Work out the finished part from the listing and answer in its coordinate system (mm). A direction names the side the tool comes from. Round coordinates to 2 decimals unless told otherwise and drop trailing zeros. Write each loop counter-clockwise with the first axis right and the second up, starting at its lowest first coordinate (ties: lowest second). Pieces come first, ordered by that corner, then holes.
1. Find section A-A (y = 0). Write down the section's boundary in (x, z), and give its area (3 significant figures).
2. Straight lines are drawn through the part: probe 1 along Y at (x, z) = (1.5, 0); probe 2 along Y at (x, z) = (0.5, -1); probe 3 along Y at (x, z) = (3.75, 0.25). For each, find the intervals that lie inside material, in ascending order.
3. Flat-ended cylindrical pins translate along their axes: pin 1 Ø2 at (x, y) = (1.5, 5.5) entering from +Z; pin 2 Ø7.5 at (y, z) = (16, -0.5) entering from -X; pin 3 Ø2 at (x, y) = (-0.5, 42) entering from -Z. Find the tip coordinate at first contact, or state that the pin passes through.
4. A tool of negligible diameter and unlimited length cuts with its end or side. For faces 3 (the face through (4, -2, -6)), 4 (the face through (-1, 20, 0)), 5 (the face through (1.8, 23.2, 3.4)), 6 (the face through (0.043, 22.839, 4.435)), 7 (the face through (0.043, 22.357, -4.476)), from which of +Z, -Z, +X, -X, +Y, -Y can it reach the whole face along a straight path? Write none if from no direction.
5. Determine the mould class of faces 1 (the face through (-1.5, 38, 0)), 2 (the face through (-4, -2, -6)) for opening direction Y: pulls with the +Y half, pulls with the -Y half, needs draft (parallel to the pull), parting line crosses it, or undercut.
6. Find section C-C (y = 21.5). Write down the section's boundary in (x, z), and give its area (3 significant figures).
7. Find section B-B (z = -1.5). Count the separate pieces of the cut face and the enclosed holes in it, and give its area (3 significant figures).
```python
from build123d import *

# Parameters (mm, degrees)
BOSS_EXTRU_1_START      = -2.0000001
BOSS_EXTRU_1_DEPTH      = 2.0000001
BOSS_EXTRU_1_START_2    = 2.0000001
BOSS_EXTRU_1_2_DEPTH    = 1.088880676
BOSS_EXTRU_1_START_3    = 3.256370695
BOSS_EXTRU_1_3_DEPTH    = 1.743629305
BOSS_EXTRU_1_START_4    = 3.172268194
BOSS_EXTRU_1_4_DEPTH    = 0.084102501
ENL_V_MAT_EXTRU_1_DEPTH = 9


with BuildPart() as part:
    # Esquisse2 → Révolution1 (revolve)
    with BuildSketch(Plane.XY, mode=Mode.PRIVATE) as r_volution1_sk:
        Polygon((2.4e-16, 6), (4, 6), (4, 7), (2.9999999999999996, 8), (-1.8e-16, 8), align=None)
    revolve(r_volution1_sk.sketch.rotate(Axis((0, 0, 0), (1, 0, 0)), 90), axis=Axis((0, 0, 0), (1, 0, 0)))



with BuildPart() as body_2:
    # Esquisse3 → Révolution2 (revolve)
    with BuildSketch(Plane.XY, mode=Mode.PRIVATE) as r_volution2_sk:
        Polygon((0, 48.99999999999999), (4.01e-15, 51), (2, 51), (4, 49.99999999999999), (4, 48.99999999999999), align=None)
    revolve(r_volution2_sk.sketch.rotate(Axis((0, 45, 0), (1, 0, 0)), 90), axis=Axis((0, 45, 0), (1, 0, 0)))


with BuildPart() as part_1:
    add(part.part)

    add(body_2.part)  # Boss.-Extru.1 merges body 2
    # Boss.-Extru.1: read off the stored shape, not the designer's step
    # Boss.-Extru.1 outline → Boss.-Extru.1 (add)
    with BuildSketch(Plane.ZY.offset(BOSS_EXTRU_1_START)):
        with BuildLine():
            ThreePointArc((-5.910337632, 5.39146632), (0, 8), (5.910337632, 5.39146632))
            Line((5.910337632, 5.39146632), (3, 39.803847577))
            ThreePointArc((3, 39.803847577), (0, 39), (-3, 39.803847577))
            Line((-3, 39.803847577), (-5.910337632, 5.39146632))
        make_face()
    extrude(amount=BOSS_EXTRU_1_DEPTH)

    # Boss.-Extru.1 2 outline → Boss.-Extru.1 2 (add)
    with BuildSketch(Plane.YZ.offset(BOSS_EXTRU_1_START_2)):
        with BuildLine():
            ThreePointArc((39.803847577, -3), (39, 0), (39.803847577, 3))
            Line((39.803847577, 3), (5.39146632, 5.910337632))
            ThreePointArc((5.39146632, 5.910337632), (8, 0), (5.39146632, -5.910337632))
            Line((5.39146632, -5.910337632), (39.803847577, -3))
        make_face()
    extrude(amount=BOSS_EXTRU_1_2_DEPTH)

    # Boss.-Extru.1 3 outline → Boss.-Extru.1 3 (cut)
    with BuildSketch(Plane(origin=(0, 0, 0), x_dir=(-0.032241294010957995, 0.9994801143396995, 0), z_dir=(0.9994801143396996, 0.032241294010957995, 0)).offset(BOSS_EXTRU_1_START_3)):
        with BuildLine():
            add(Edge.make_bspline(
                [(5.142379796, -5.922750354), (12.17659734275441, -2.94e-15), (5.142379796, 5.922750354)],
                knots=[5.412727934893089, 5.412727934893089, 5.412727934893089, 7.153642679466084, 7.153642679466084, 7.153642679466084], degree=2, weights=[1, 0.6444768969331849, 1]))
            Line((5.142379796, -5.922750354), (39.719507575, -3))
            add(Edge.make_bspline(
                [(39.719507575, -3), (39.4087631690425, -2.4620547166991407), (39.162117173894764, -1.8742292038542891), (38.995705810616975, -1.2534964190781404), (38.91524187122639, -0.6211657082460426), (38.91524187122635, 0.6211657082460548), (38.99570581061705, 1.2534964190781592), (39.16211717389469, 1.8742292038543251), (39.40876316904256, 2.46205471669918), (39.719507575, 3)],
                knots=[3.141592653589793, 3.141592653589793, 3.141592653589793, 3.141592653589793, 3.141592653589793, 3.141592653589793, 3.665191429188086, 3.665191429188086, 3.665191429188086, 3.665191429188086, 4.188790204786387, 4.188790204786387, 4.188790204786387, 4.188790204786387, 4.188790204786387, 4.188790204786387], degree=5, weights=[1, 0.9999999999999991, 0.9995355802743678, 0.9995355802743658, 1.0000000000000004, 0.9999999999999986, 0.9995355802743691, 0.9995355802743657, 1.0000000000000004, 1]))
            Line((39.719507575, 3), (5.142379796, 5.922750354))
        make_face()
    extrude(amount=BOSS_EXTRU_1_3_DEPTH, mode=Mode.SUBTRACT)

    # Boss.-Extru.1 4 outline → Boss.-Extru.1 4 (add)
    with BuildSketch(Plane(origin=(0, 0, 0), x_dir=(-0.032241294010957995, 0.9994801143396995, 0), z_dir=(0.9994801143396996, 0.032241294010957995, 0)).offset(BOSS_EXTRU_1_START_4)):
        with BuildLine():
            add(Edge.make_bspline(
                [(5.142379796, -5.922750354), (12.17659734275441, -2.94e-15), (5.142379796, 5.922750354)],
                knots=[5.412727934893089, 5.412727934893089, 5.412727934893089, 7.153642679466084, 7.153642679466084, 7.153642679466084], degree=2, weights=[1, 0.6444768969331849, 1]))
            Line((5.142379796, -5.922750354), (39.719507575, -3))
            add(Edge.make_bspline(
                [(39.719507575, -3), (39.4087631690425, -2.4620547166991407), (39.162117173894764, -1.8742292038542891), (38.995705810616975, -1.2534964190781404), (38.91524187122639, -0.6211657082460426), (38.91524187122635, 0.6211657082460548), (38.99570581061705, 1.2534964190781592), (39.16211717389469, 1.8742292038543251), (39.40876316904256, 2.46205471669918), (39.719507575, 3)],
                knots=[3.141592653589793, 3.141592653589793, 3.141592653589793, 3.141592653589793, 3.141592653589793, 3.141592653589793, 3.665191429188086, 3.665191429188086, 3.665191429188086, 3.665191429188086, 4.188790204786387, 4.188790204786387, 4.188790204786387, 4.188790204786387, 4.188790204786387, 4.188790204786387], degree=5, weights=[1, 0.9999999999999991, 0.9995355802743678, 0.9995355802743658, 1.0000000000000004, 0.9999999999999986, 0.9995355802743691, 0.9995355802743657, 1.0000000000000004, 1]))
            Line((39.719507575, 3), (5.142379796, 5.922750354))
        make_face()
    extrude(amount=BOSS_EXTRU_1_4_DEPTH)

    # Esquisse6 → Enlèv. mat.-Extru.1 (cut)
    with BuildSketch(Plane(origin=(10, 0, 0), x_dir=(0, 0, -1), z_dir=(1, 0, 0))):
        with BuildLine():
            Line((4.7185213239125305, 7.617327682628814), (2.121151849996758, 38.329114389434075))
            ThreePointArc((2.121151849996758, 38.329114389434075), (1.0732662125583343, 38.082767920838506), (1.29e-15, 37.999999999999986))
            ThreePointArc((1.29e-15, 37.999999999999986), (-1.0732662125583345, 38.08276792083852), (-2.12115184999676, 38.32911438943409))
            Line((-2.12115184999676, 38.32911438943409), (-4.7185213239117045, 7.617327682628745))
            add(Edge.make_bspline(
                [(-4.7185213239117045, 7.617327682628745), (-4.011984255343939, 8.070257956932029), (-3.261550361542695, 8.410740591888102), (-2.2711967086518885, 8.702341470829111), (-2.0704598676815316, 8.75383204519997), (-1.6635130029960632, 8.842792898029453), (-1.456446032141917, 8.880350619711338), (-0.8364313606849374, 8.969908948596256), (-0.00941084225722518, 9.029205401703816), (0.818259414860091, 8.971660679545408), (1.646265253396883, 8.853769039344968), (2.0556953800959668, 8.76494999754429), (2.850690444417165, 8.532525136333405), (3.23863975479659, 8.388601680371798), (3.9952504696443585, 8.044777052176354), (4.365252036804486, 7.8437933023834185), (4.7185213239125305, 7.617327682628814)],
                knots=[0, 0, 0, 0, 0.24999999999999978, 0.24999999999999978, 0.31249999999999983, 0.31249999999999983, 0.3749999999999999, 0.3749999999999999, 0.4999999999999999, 0.6249999999999999, 0.6249999999999999, 0.7499999999999999, 0.7499999999999999, 0.8749999999999999, 0.8749999999999999, 1, 1, 1, 1], degree=3))
        make_face()
    extrude(amount=-ENL_V_MAT_EXTRU_1_DEPTH, mode=Mode.SUBTRACT)

    # Symétrie10: part across plane


with BuildPart() as part_2:
    add(part_1.part)
    add(part_1.part.mirror(Plane(origin=(0, 0, 0), x_dir=(0, 0, 1), z_dir=(1, 0, 0))))


solid = part_2.part
```
Worked answers:
1. outline: (-4, -7) - (-3, -8) - (3, -8) - (4, -7) - (4, -6) - (-4, -6) - close; (-4, 6) - (4, 6) - (4, 7) - (3, 8) - (-3, 8) - (-4, 7) - close
1. area: 30.0 mm2
2. probe 1: y = -8 to -6, 6 to 9, 38 to 41, 49 to 51
2. probe 2: y = -7.94 to -5.92, 5.92 to 41.13, 48.87 to 50.92
2. probe 3: y = -7.25 to -5.99, 5.99 to 7.25, 39.88 to 41.01, 48.99 to 50.12
3. pin 1: stops at z = 6.61
3. pin 2: stops at x = -2.78
3. pin 3: stops at z = -5.66
4. face 3: +Z, -Z, +X, +Y, -Y
4. face 4: -X
4. face 5: +X
4. face 6: +Z, +X, -X
4. face 7: -Z, +X, -X
5. face 1: undercut
5. face 2: needs draft
6. outline: (-2.56, -4.55) - (2.56, -4.55) - (2.56, -3.54) - (1, -3.54) - (1, 3.54) - (2.56, 3.54) - (2.56, 4.55) - (-2.56, 4.55) - (-2.56, 3.54) - (-1, 3.54) - (-1, -3.54) - (-2.56, -3.54) - close
6. area: 24.5 mm2
7. separate pieces: 3
7. enclosed holes: 0
7. area: 129 mm2
